from build123d import *

# Parameters (mm, degrees)
F1_W     = 54
F1_H     = 4
F2_DEPTH = 5
F4_DEPTH = 5
F6_DEPTH = 5


with BuildPart() as f2:
    # F1 (on Front) → F2 (new body, symmetric)
    with BuildSketch(Plane.XZ):
        with Locations((0, 24.4391597784)):
            Rectangle(F1_W, F1_H)
    extrude(amount=F2_DEPTH, both=True)

    # F5: F4 across plane


with BuildPart() as f4:
    # F3 (on Front) → F4 (new body, symmetric)
    with BuildSketch(Plane.XZ):
        Polygon((21.6551174292, 34.4391597784), (20.4551174292, 24.4391597784), (21.6551174292, 14.4391597784), (23.6551174292, 14.4391597784), (24.8551174292, 24.4391597784), (23.6551174292, 34.4391597784), align=None)
    extrude(amount=F4_DEPTH, both=True)


with BuildPart() as f2_1:
    add(f2.part)
    add(f4.part.mirror(Plane.YZ))


    add(f4.part)  # F6 merges F4
    # F0 (on Front) → F6 (join, symmetric)
    with BuildSketch(Plane.XZ):
        with BuildLine():
            Line((-21, 26.4391597784), (21, 26.4391597784))
            Line((21, 26.4391597784), (21, 28.9798478681))
            add(Edge.make_bspline(
                [(-21, 28.9798478681), (-19.5953512364, 28.8401652252), (-17.391429418, 29.8376339387), (-13.9476569454, 32.6070199787), (-10.5904127723, 35.42087783), (-7.0658407923, 37.3677794905), (-3.5015046033, 38.199162892), (-0.0004836835, 38.5579308119), (3.5247350414, 38.2002323502), (7.084375424, 37.3668707381), (10.6175923145, 35.4245267912), (13.9608785638, 32.5811894464), (17.4960225284, 29.8837543114), (19.7866070593, 28.8401652252), (21, 28.9798478681)],
                knots=[0, 0, 0, 0, 0.0806013739, 0.1686553866, 0.2573747863, 0.3413343067, 0.4214474157, 0.5001651337, 0.5791215884, 0.6592349037, 0.7431945127, 0.831913137, 0.921023509, 1, 1, 1, 1], degree=3))
            Line((-21, 28.9798478681), (-21, 26.4391597784))
        make_face()
    extrude(amount=F6_DEPTH, both=True)


solid = f2_1.part
Design review of the part built by this model. Coordinates are the model's own, in mm. A direction names the side the tool comes from. Coordinates: 2 decimals unless noted, no trailing zeros. Order: outer loops, then holes, each group sorted by start corner. A loop starts at its lowest first (then second) coordinate and runs counter-clockwise, first axis right, second up. Notation, with made-up numbers: (21.25, -32) -> (46.25, -32) arc R21 cw to (46.25, -25) -> close; hole circle Ø2 at (34.25, -3.5). An arc over 180 degrees is marked (long way). Use one line per item in the form item = value. Start each with the question number.
(1) For probe 1 along X at (y, z) = (0.75, 32.5); probe 2 along X at (y, z) = (-1.5, 31.75); probe 3 along Z at (x, y) = (-22.5, 0.5), list the stretches that pass through material, from the lowest coordinate up.
(2) Add section C-C on x = -23. State the section outline as (y, z) points, plus the area to 3 significant figures.
(3) For faces 1 (the flat face through (-23, 0, 34.439)), 2 (the flat face through (-26, 0, 22.439)), 3 (the flat face through (26, 0, 22.439)), 4 (the flat face through (-21.332, -0.07, 31.748)), 5 (the flat face through (-21.168, -0.07, 18.495)), list the 3-axis set-ups (+Z, -Z, +X, -X, +Y, -Y) from which the entire face can be reached by the end or side of a thin tool; tool diameter is ignored.
(4) Add section D-D on z = 30.5. Give the number of separate pieces and of enclosed holes in the cut face, plus the area to 3 significant figures.
(5) Add section A-A on z = 18.5. State the section outline as (x, y) points.
(6) The part is to be moulded in two halves that separate along X. For faces 6 (the flat face through (-24.13, -0.07, 18.38)), 7 (the flat face through (27, 0, 24)), 8 (the flat face through (0, 0, 22.439)), 9 (the flat face through (0, 5, 29)), say which applies: +X half, -X half, draft (parallel to the pull), parting line (faces both ways), or undercut.
(7) Insertion check: pin 1 (1.9 mm diameter, centred on x = -26, y = -0.5, fed in from +Z); pin 2 (1.5 mm diameter, centred on x = 18.5, y = 3.5, fed in from -Z); pin 3 (0.6 mm diameter, centred on x = 22, y = -1, fed in from +Z). Each pin has a flat end and moves straight along its axis. Give the tip position at first contact, or say it passes through.
(8) Add section B-B on z = 21. State the section outline as (x, y) points.
Answer block:
q1.probe_1 = -23.89 to -21.42, -14.1 to 14.13, 21.42 to 23.89
q1.probe_2 = -23.98 to -21.33, -15.03 to 15.08, 21.33 to 23.98
q1.probe_3 = 14.44 to 34.44
q2.outline = (-5, 14.44) -> (5, 14.44) -> (5, 34.44) -> (-5, 34.44) -> close
q2.area = 200 mm²
q3.face_1 = +Z, -X, +Y, -Y
q3.face_2 = -Z, -X, +Y, -Y
q3.face_3 = -Z, +X, +Y, -Y
q3.face_4 = +Z, +Y, -Y
q3.face_5 = -Z, +Y, -Y
q4.separate_pieces = 3
q4.enclosed_holes = 0
q4.area = 394 mm²
q5.outline = (-24.14, -5) -> (-21.17, -5) -> (-21.17, 5) -> (-24.14, 5) -> close; (21.17, -5) -> (24.14, -5) -> (24.14, 5) -> (21.17, 5) -> close
q6.face_6 = -X half
q6.face_7 = +X half
q6.face_8 = undercut
q6.face_9 = draft
q7.pin_1 = 26.44
q7.pin_2 = 22.44
q7.pin_3 = 34.44
q8.outline = (-24.44, -5) -> (-20.87, -5) -> (-20.87, 5) -> (-24.44, 5) -> close; (20.87, -5) -> (24.44, -5) -> (24.44, 5) -> (20.87, 5) -> close
